```python
from build123d import *

# Parameters (mm, degrees)
RESSALTO_EXTRUS_O1_DEPTH   = 285
CORTE_EXTRUS_O1_DEPTH      = 1
CORTE_EXTRUS_O1_DEPTH_BACK = 286
ESBO_O3_R                  = 2.25
CORTE_EXTRUS_O2_DEPTH      = 130
ESBO_O4_R                  = 1.645507678
CORTE_EXTRUS_O3_DEPTH      = 15
ESBO_O5_R                  = 3.5
CORTE_EXTRUS_O4_DEPTH      = 10
CORTE_EXTRUS_O5_START      = -10
ESBO_O6_R                  = 4.5
CORTE_EXTRUS_O5_DEPTH      = 120
ESBO_O7_W                  = 1.5
ESBO_O7_H                  = 2
CORTE_EXTRUS_O6_DEPTH      = 124.176451884
CORTE_EXTRUS_O6_DEPTH_BACK = 1
ESBO_O8_R                  = 1.25
CORTE_EXTRUS_O7_DEPTH      = 10


with BuildPart() as part:
    # Esboço1 → Ressalto-extrusão1 (new body)
    with BuildSketch(Plane.XY):
        Polygon((0, 75), (135.77, 75), (135.77, 0), (132.504208406, 0), (130.985, 59), (122.235, 59), (120.715791594, 0), (119.454208406, 0), (117.935, 59), (109.185, 59), (107.665791594, 0), (106.404208406, 0), (104.885, 59), (96.135, 59), (94.615791594, 0), (93.354208406, 0), (91.835, 59), (83.085, 59), (81.565791594, 0), (80.304208406, 0), (78.785, 59), (70.035, 59), (68.515791594, 0), (67.254208406, 0), (65.735, 59), (56.985, 59), (55.465791594, 0), (54.204208406, 0), (52.685, 59), (43.935, 59), (42.415791594, 0), (41.154208406, 0), (39.635, 59), (30.885, 59), (29.365791594, 0), (28.104208406, 0), (26.585, 59), (17.835, 59), (16.315791594, 0), (15.054208406, 0), (13.535, 59), (4.785, 59), (3.265791594, 0), (0, 0), align=None)
    extrude(amount=RESSALTO_EXTRUS_O1_DEPTH)

    # Esboço2 → Corte-extrusão1 (cut, two sides)
    with BuildSketch(Plane(origin=(0, 0, 0), x_dir=(-1, 0, 0), z_dir=(0, 0, -1))) as corte_extrus_o1_sk:
        Polygon((-21.831152423, 75), (-20.831152423, 73.267949192), (-19.099101615, 74.267949192), (-18.099101615, 72.535898385), (-19.831152423, 71.535898385), (-12.593548116, 59), (-12.593548116, -2.874547604), (9.502168499, -2.874547604), (9.502168499, 75), align=None)
        Polygon((-113.938847577, 75), (-114.938847577, 73.267949192), (-111.907758664, 71.517949192), (-112.907758664, 69.785898385), (-115.938847577, 71.535898385), (-123.176451884, 59), (-123.176451884, -2.874547604), (-142.207346128, -2.874547604), (-142.207346128, 78.515038313), (-113.938847577, 78.515038313), align=None)
    extrude(amount=CORTE_EXTRUS_O1_DEPTH, mode=Mode.SUBTRACT)
    extrude(corte_extrus_o1_sk.sketch, amount=-CORTE_EXTRUS_O1_DEPTH_BACK, mode=Mode.SUBTRACT)

    # Esboço3 → Corte-extrusão2 (cut)
    with BuildSketch(Plane(origin=(117.930088325, 68.08696824, 0), x_dir=(0, 0, -1), z_dir=(0.866025404, 0.5, 0))):
        with Locations((-275, -4.017518505)):
            Circle(ESBO_O3_R)
        with Locations((-45, -4.017518505)):
            Circle(ESBO_O3_R)
    extrude(amount=-CORTE_EXTRUS_O2_DEPTH, mode=Mode.SUBTRACT)

    # Esboço4 → Corte-extrusão3 (cut)
    with BuildSketch(Plane(origin=(-16.102588325, 9.296833704, 0), x_dir=(0, 0, 1), z_dir=(-0.866025404, 0.5, 0))):
        with Locations((45, 63.867481495)):
            Circle(ESBO_O4_R)
        with Locations((275, 63.867481495)):
            Circle(ESBO_O4_R)
    extrude(amount=-CORTE_EXTRUS_O3_DEPTH, mode=Mode.SUBTRACT)

    # Esboço5 → Corte-extrusão4 (cut)
    with BuildSketch(Plane(origin=(0, 0, 0), x_dir=(-1, 0, 0), z_dir=(0, 0, -1))):
        with Locations((-67.885, 49.767603925)):
            Circle(ESBO_O5_R)
    extrude(amount=-CORTE_EXTRUS_O4_DEPTH, mode=Mode.SUBTRACT)

    # Esboço6 → Corte-extrusão5 (cut)
    with BuildSketch(Plane(origin=(117.930088325, 68.08696824, 0), x_dir=(0, 0, -1), z_dir=(0.866025404, 0.5, 0)).offset(CORTE_EXTRUS_O5_START)):
        with Locations((-275, -4.017518505)):
            Circle(ESBO_O6_R)
        with Locations((-45, -4.017518505)):
            Circle(ESBO_O6_R)
    extrude(amount=-CORTE_EXTRUS_O5_DEPTH, mode=Mode.SUBTRACT)

    # Esboço7 → Corte-extrusão6 (cut, two sides)
    with BuildSketch(Plane(origin=(0, 36.48769631, 0), x_dir=(0, 0, -1), z_dir=(1, 0, 0))) as corte_extrus_o6_sk:
        with Locations((-284.25, 35.51230369)):
            Rectangle(ESBO_O7_W, ESBO_O7_H)
    extrude(amount=CORTE_EXTRUS_O6_DEPTH, mode=Mode.SUBTRACT)
    extrude(corte_extrus_o6_sk.sketch, amount=-CORTE_EXTRUS_O6_DEPTH_BACK, mode=Mode.SUBTRACT)

    # Esboço8 → Corte-extrusão7 (cut)
    with BuildSketch(Plane.XY.offset(285)):
        with Locations((37.885, 69.5)):
            Circle(ESBO_O8_R)
        with Locations((97.885, 69.5)):
            Circle(ESBO_O8_R)
    extrude(amount=-CORTE_EXTRUS_O7_DEPTH, mode=Mode.SUBTRACT)


solid = part.part
```
Can you work these out from the model? Positions are in its coordinate system, mm. A direction names the side the tool comes from. Give positions to 0.01 mm unless a question says otherwise; leave off trailing zeros. One line per item, written item: value.
Q1. For P1, Ø4.5, axis at x = 22, z = 170.5, coming from the -Y side; P2, Ø0.6, axis at x = 116, y = 71.5, coming from the +Z side; P3, Ø12, axis at y = 12.5, z = 142.5, coming from the -X side; P4, Ø4, axis at x = 50, y = 53.5, coming from the -Z side, each with a flat end and sliding along its axis, tell me the tip position at first contact or that it passes through.
Results found:
P1: stops at y = 59
P2: stops at z = 283.5
P3: stops at x = 14.58
P4: passes through
Q2. We'd pull the mould along X, two halves only. Please class faces 3 (the face through (22, 59, 141)), 4 (the face through (119.507, 65.356, 140.505)): +X half, -X half, draft (parallel to the pull), parting line (faces both ways), or undercut.
Results found:
face 3: undercut
face 4: +X half
Q3. Which directions (+Z, -Z, +X, -X, +Y, -Y) give clear straight access to the entire face, cutting with the end or side of a thin tool? Please do faces 1 (the face through (40.839, 22.666, 271.864)), 2 (the face through (74, 59, 141)).
Results found:
face 1: none
face 2: +Z, -Z, -Y
Q4. Please list where these lines run through material, in increasing order: line 1 (Z direction, x = 27, y = 58); line 2 (Y direction, x = 70.5, z = 160); line 3 (X direction, y = 69.5, z = 277.5) (3 decimals). Write a range as [from, to].
Results found:
line 1: z = [0, 43.36], [46.64, 273.36], [276.64, 285]
line 2: y = [59, 75]
line 3: x = [18.656, 36.635], [39.135, 96.635], [99.135, 117.114]
